Source: CAD feature listing. Evaluate the final solid. Frame: model axes, mm. Coordinates: 2 decimals unless noted, no trailing zeros. Write each loop counter-clockwise with the first axis right and the second up, starting at its lowest first coordinate (ties: lowest second). Pieces come first, ordered by that corner, then holes. Notation, with made-up numbers: M 79.5,36 L 119.5,36 A18 cw 119.5,45 Z; hole C 54.25,-11 d10. An arc over 180 degrees is marked long. Write item = value, one per line. Start each with the question number.
1. Section query A-A (z = 1). Output: boundary loops of the cut face in (x, y), then the cut area to 3 significant figures.
2. Pin query (flat end, axial travel): pin 1 Ø8 at (x, z) = (-7.5, -7.5) entering from -Y; pin 2 Ø5 at (x, z) = (-0.5, -6) entering from -Y; pin 3 Ø6 at (x, z) = (14, 1.5) entering from +Y. Return the tip coordinate at first contact, or that it passes through.
3. Line query: line 1 along Y through (x, z) = (17.5, -11.25); line 2 along Y through (x, z) = (-18, -3). Output: solid intervals per line, ascending.
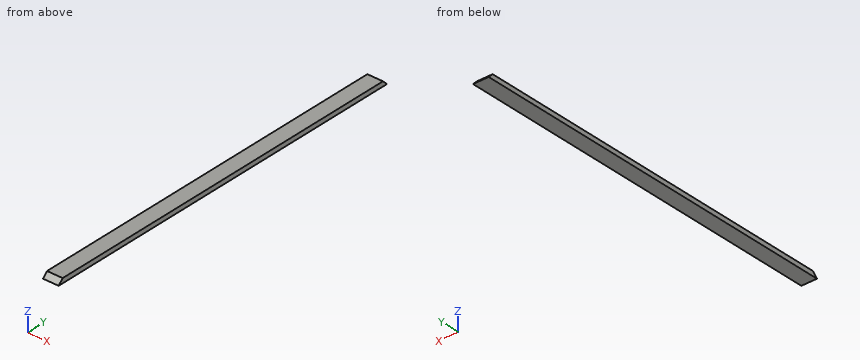
```python
from build123d import *

# Parameters (mm, degrees)
F0_W     = 63.5
F0_H     = 38.1
F1_DEPTH = 1549.4
F3_DEPTH = 76.2
F4_W     = 63.5
F4_H     = 19.05
F5_DEPTH = 1549.401


with BuildPart() as f1:
    # F0 (on Front) → F1 (new body)
    with BuildSketch(Plane.XZ):
        with Locations((5.109261, 4.715717)):
            Rectangle(F0_W, F0_H)
    extrude(amount=F1_DEPTH)

    # F2 (on face) → F3 (cut)
    with BuildSketch(Plane.YZ.offset(36.859261)):
        Polygon((-1549.4, 23.765717), (-1549.4, -14.334283), (-1511.3, 23.765717), align=None)
        Polygon((-38.1, 23.765717), (0, -14.334283), (0, 23.765717), align=None)
    extrude(amount=-F3_DEPTH, mode=Mode.SUBTRACT)

    # F4 (on Front) → F5 (cut, through all)
    with BuildSketch(Plane.XZ):
        with Locations((5.109261, 14.240717)):
            Rectangle(F4_W, F4_H)
    extrude(amount=F5_DEPTH, mode=Mode.SUBTRACT)


solid = f1.part
```
Results are:
q1.outline = M -26.64,-1534.07 L 36.86,-1534.07 L 36.86,-15.33 L -26.64,-15.33 Z
q1.area = 96,400 mm^2
q2.pin_1 = -1546.57
q2.pin_2 = -1543.57
q2.pin_3 = -12.83
q3.line_1 = -1546.32 to -3.08
q3.line_2 = -1538.07 to -11.33
